The model under review builds one solid part; all positions refer to its coordinate system, in mm. Face numbers are marked on the shaded views. A direction names the side the tool comes from. Coordinates: 2 decimals unless noted, no trailing zeros. Order: outer loops, then holes, each group sorted by start corner. A loop starts at its lowest first (then second) coordinate and runs counter-clockwise, first axis right, second up. Notation, with made-up numbers: M 47,7.5 L 56,7.5 A30 cw 56,45.5 Z; hole C 79.25,21 d7. An arc over 180 degrees is marked long. Answer in a Markdown table with one row per item.
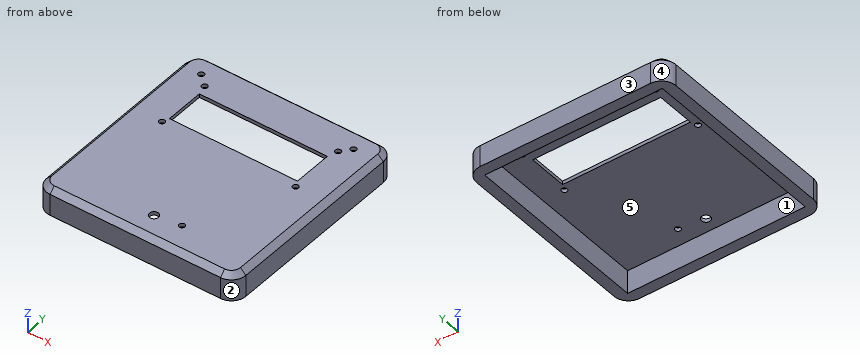
Autodesk Inventor part; units mm, degrees
ref_plane "YZ Plane" through (0, 0, 0) normal (1, 0, 0) x (0, 1, 0)
ref_plane "XZ Plane" through (0, 0, 0) normal (0, 1, 0) x (-1, 0, 0)
ref_plane "XY Plane" through (0, 0, 0) normal (0, 0, 1) x (1, 0, 0)
sketch "Sketch1" plane through (0, 0, 0) normal (0, 0, 1) x (1, 0, 0)
  line L0 (0, 103.81) -> (0, 0)
  line L1 (99.04, 103.81) -> (0, 103.81)
  line L2 (99.04, 0) -> (99.04, 103.81)
  circle A0 centre (91.5302, 97.8155) radius 1.6
  circle A1 centre (6.3166, 98.2023) radius 1.6
  circle A2 centre (63.7434, 9.4559) radius 1.6
  line L3 (-2.8877, 39.67) -> (-2.8877, 25.07)
  line L4 (18.04, 39.67) -> (-2.8877, 39.67)
  line L5 (-2.8877, 25.07) -> (18.04, 25.07)
  line L6 (5.99, 20.97) -> (-0.5, 20.97)
  line L7 (-0.5, 20.97) -> (-0.5, 9.286)
  line L8 (-0.5, 9.286) -> (5.99, 9.286)
  line L9 (5.99, 9.286) -> (5.99, 20.97)
  line L10 (18.04, 25.07) -> (18.04, 39.67)
  line L11 (0, 0) -> (99.04, 0)
  line L12 (-2, 105.81) -> (-2, -2)
  line L13 (-2, -2) -> (101.04, -2)
  line L14 (101.04, -2) -> (101.04, 105.81)
  line L15 (101.04, 105.81) -> (-2, 105.81)
  line L16 (-6, 109.81) -> (-6, -6)
  line L17 (-6, -6) -> (105.04, -6)
  line L18 (105.04, -6) -> (105.04, 109.81)
  line L19 (105.04, 109.81) -> (-6, 109.81)
  circle A3 centre (49.53, 7.62) radius 1.55
  point P0 (0, 20.97)
  point P1 (0, 9.286)
  dimension "d0" = 2
  dimension "d1" = 4
extrude "Extrusion3" add sketch "Sketch1" against normal blind 15 contours L0 L4 L12 L15 L14 L13 L5 L6 L7 L8 L11 L2 L1 | L0 L5 L12 L4 | L12 L5 L3 L4 | L0 L8 L7 L6 | L19 L18 L17 L16
extrude "Extrusion4" add sketch "Sketch1" against normal blind 2 contours L1 L2 L11 L0 L8 L9 L6 L5 L10 L4 | L4 L10 L5 L0 | L6 L9 L8 L0 | A3
fillet "Fillet2" radius 8 4 edges at (105.04, -6, -7.5) (-6, -6, -7.5) (-6, 109.81, -7.5) (105.04, 109.81, -7.5)
chamfer "Chamfer2" distance 3 angle 45 8 edges at (-6, 51.905, 0) (-3.6569, -3.6569, 0) (49.52, -6, 0) (102.6969, -3.6569, 0) (105.04, 51.905, 0) (102.6969, 107.4669, 0) (49.52, 109.81, 0) (-3.6569, 107.4669, 0)
sketch "Sketch2" plane through (0, 0, 0) normal (0, 0, 1) x (1, 0, 0)
  circle A0 centre (49.53, 7.62) radius 1.55
  circle A1 centre (49.53, 7.62) radius 2.5
  point P0 (0, 0)
  dimension "d18" = 5
extrude "Extrusion5" cut sketch "Sketch2" against normal blind 2 contours A0 | A1
sketch "Sketch3" plane through (0, 0, 0) normal (0, 0, 1) x (1, 0, 0)
  line L0 (9.9957, 94.7225) -> (9.9957, 59.1825)
  line L1 (9.9957, 59.1825) -> (90.0757, 59.1825)
  line L2 (90.0757, 59.1825) -> (90.0757, 94.7225)
  line L3 (90.0757, 94.7225) -> (9.9957, 94.7225)
  circle A0 centre (12.6104, 92.4416) radius 1.595
  circle A1 centre (87.094, 61.4588) radius 1.595
  line L4 (13.9957, 86.8134) -> (13.9957, 65.1061)
  line L5 (85.3757, 86.8134) -> (13.9957, 86.8134)
  line L6 (85.3757, 65.1061) -> (85.3757, 86.8134)
  line L7 (13.9957, 65.1061) -> (85.3757, 65.1061)
  circle A2 centre (87.094, 92.4416) radius 1.595
  circle A3 centre (12.6104, 61.4588) radius 1.595
  line L8 (49.6857, 86.8134) -> (49.6857, 75.9598)
  line L9 (2, 106.81) -> (97.04, 106.81)
  point P0 (0, 0)
  point P1 (55.3023, 77.61)
extrude "Extrusion6" cut sketch "Sketch3" against normal blind 2 contours A0 | A1 | L5 L6 L7 L4 | A2 | A3
properties part number "Tampa"
(1) To check wall thickness, follow line 1 (Y direction, x = 95, z = -6); line 2 (X direction, y = 92, z = -14); line 3 (Z direction, x = 61, y = 88.5). State the ranges of each line that lie inside material, in increasing order. Write a range as [from, to].
Report:
| item | result |
|---|---|
| line 1 | [-6, 0], [103.81, 109.81] |
| line 2 | [-6, 0], [99.04, 105.04] |
| line 3 | [-2, 0] |
(2) Take a section at A-A (y = 84). Write out the cut boundary in (x, z).
Report:
| item | result |
|---|---|
| outline | M -6,-15 L 0,-15 L 0,-2 L 14,-2 L 14,0 L -3,0 L -6,-3 Z; M 85.38,-2 L 99.04,-2 L 99.04,-15 L 105.04,-15 L 105.04,-3 L 102.04,0 L 85.38,0 Z |
(3) Insertion check: P1, Ø4, axis at x = 63.74, y = 9.46, coming from the -Z side; P2, Ø3, axis at x = 91.53, y = 97.82, coming from the +Z side; P3, Ø1.6, axis at y = 80, z = -1.5, coming from the +X side; P4, Ø1, axis at x = 51.5, z = -1, coming from the -Y side. Each pin has a flat end and moves straight along its axis. Give the tip position at first contact, or say it passes through.
Report:
| item | result |
|---|---|
| P1 | z = -2 |
| P2 | through |
| P3 | x = 104.34 |
| P4 | y = -4.5 |
(4) Take a section at D-D (x = 70). Write out the cut boundary in (y, z), then the cut area to 3 significant figures.
Report:
| item | result |
|---|---|
| outline | M -6,-15 L 0,-15 L 0,-2 L 65.11,-2 L 65.11,0 L -3,0 L -6,-3 Z; M 86.81,-2 L 103.81,-2 L 103.81,-15 L 109.81,-15 L 109.81,-3 L 106.81,0 L 86.81,0 Z |
| area | 335 mm^2 |
(5) The part is to be moulded in two halves that separate along X. For the marked faces 3, 4 and 5, say which applies: +X half, -X half, draft (parallel to the pull), parting line (faces both ways), or undercut.
Report:
| item | result |
|---|---|
| face 3 | draft |
| face 4 | -X half |
| face 5 | undercut |
(6) Take a section at C-C (x = 49.53). Write out the cut boundary in (y, z), then the cut area to 3 significant figures.
Report:
| item | result |
|---|---|
| outline | M -6,-15 L 0,-15 L 0,-2 L 5.12,-2 L 5.12,0 L -3,0 L -6,-3 Z; M 10.12,-2 L 65.11,-2 L 65.11,0 L 10.12,0 Z; M 86.81,-2 L 103.81,-2 L 103.81,-15 L 109.81,-15 L 109.81,-3 L 106.81,0 L 86.81,0 Z |
| area | 325 mm^2 |
(7) Machinability: for the marked faces 1 and 2, which of the approach directions +Z, -Z, +X, -X, +Y, -Y give a long, thin tool a straight path to every point of the face, cutting with its end or side? Answer none if there is none.
Report:
| item | result |
|---|---|
| face 1 | -Z |
| face 2 | +Z, -Z, +X, -Y |
(8) Take a section at B-B (z = -9.25). Write out the cut boundary in (x, y).
Report:
| item | result |
|---|---|
| outline | M -6,2 A8 ccw 2,-6 L 97.04,-6 A8 ccw 105.04,2 L 105.04,101.81 A8 ccw 97.04,109.81 L 2,109.81 A8 ccw -6,101.81 Z; hole M 0,0 L 99.04,0 L 99.04,103.81 L 0,103.81 Z |
